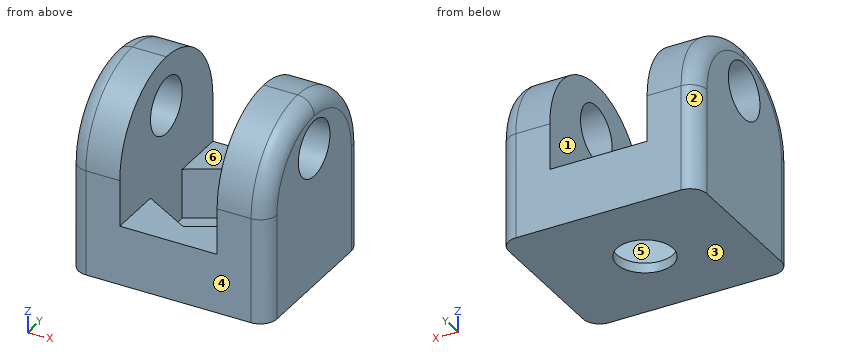
```python
from build123d import *

# Parameters (mm, degrees)
F0_R     = 1.7
F5_DEPTH = 0.6
F6_DEPTH = 3.6
F7_DEPTH = 11.4
F8_D     = 3.4
F8_DEPTH = 5
F8_START = 1
F8_TIP   = 1.0214630523
F9_D     = 3.4
F9_DEPTH = 5
F9_START = 1
F9_TIP   = 1.0214630523
F10_R    = 4.99999
F11_R    = 1


# Not quite as in the source:
# - a fillet or chamfer is up to 0.001 mm smaller than in the source, because OpenCascade refuses the exact size


with BuildPart() as f5:
    # F0 (on Top) → F5 (new body)
    with BuildSketch(Plane.XY):
        Polygon((0, 3.4), (-2.9444863729, 1.7), (-2.9444863729, -1.7), (0, -3.4), (2.9444863729, -1.7), (2.9444863729, 1.7), align=None)
        Circle(F0_R, mode=Mode.SUBTRACT)
    extrude(amount=F5_DEPTH)

    # F0 (on Top) → F6 (join)
    with BuildSketch(Plane.XY):
        Polygon((2.9444863729, 5), (-2.9444863729, 5), (-2.9444863729, 1.7), (0, 3.4), (2.9444863729, 1.7), align=None)
        Polygon((-2.9444863729, -1.7), (-2.9444863729, -5), (2.9444863729, -5), (2.9444863729, -1.7), (0, -3.4), align=None)
    extrude(amount=F6_DEPTH)

    # F0 (on Top) → F7 (join)
    with BuildSketch(Plane.XY):
        Polygon((-2.9444863729, 5), (-6, 5), (-6, -5), (-2.9444863729, -5), (-2.9444863729, -1.7), (-2.9444863729, 1.7), align=None)
        Polygon((6, 5), (2.9444863729, 5), (2.9444863729, 1.7), (2.9444863729, -1.7), (2.9444863729, -5), (6, -5), align=None)
    extrude(amount=F7_DEPTH)

    # F8
    # its depths count from where the whole tool has entered the part; down to there all is cleared
    with Locations(Plane(origin=(-7, 0, 0), x_dir=(0, 1, 0), z_dir=(-1, 0, 0)).offset(-F8_START)):
        with Locations((0, -8.4)):
            Hole(F8_D / 2, depth=F8_DEPTH)
            with Locations((0, 0, -(F8_DEPTH + F8_TIP / 2))):  # 118° drill point
                Cone(0, F8_D / 2, F8_TIP, mode=Mode.SUBTRACT)

    # F9
    # its depths count from where the whole tool has entered the part; down to there all is cleared
    with Locations(Plane.YZ.offset(7).offset(-F9_START)):
        with Locations((0, 8.4)):
            Hole(F9_D / 2, depth=F9_DEPTH)
            with Locations((0, 0, -(F9_DEPTH + F9_TIP / 2))):  # 118° drill point
                Cone(0, F9_D / 2, F9_TIP, mode=Mode.SUBTRACT)

    # F10 (radius 5 in the source; OpenCascade refuses exactly that, so slightly less here)
    f10_edges = [f5.edges().sort_by_distance(p)[0] for p in [
        (-4.472243, -5, 11.4),
        (-4.472243, 5, 11.4),
        (4.472243, 5, 11.4),
        (4.472243, -5, 11.4),
    ]]
    fillet(f10_edges, radius=F10_R)

    # F11
    f11_edges = [f5.edges().sort_by_distance(p)[0] for p in [
        (6, 3.535537, 9.935537),
        (-6, 3.535537, 9.935537),
    ]]
    fillet(f11_edges, radius=F11_R)


solid = f5.part
```
The listing builds one solid part. Answer for the finished solid, in the listing's coordinates (mm). Face numbers are marked on the shaded views. A direction names the side the tool comes from. Round coordinates to 2 decimals unless told otherwise and drop trailing zeros. Loops run counter-clockwise (first coordinate to the right, second up) from the corner with the lowest first, then second, coordinate; pieces in that order, holes last.
Q1. Section B-B, the plane z = 5.75 is taken. Determine the outline of the cut face in (x, y).
Q2. Section C-C, the plane x = -0.25 is taken. Determine the outline of the cut face in (y, z), then the cut area to 3 significant figures.
Q3. Find the intervals of material crossed by line 1 (X direction, y = 1.5, z = 1.5); line 2 (Y direction, x = 0, z = 0.35); line 3 (Z direction, x = 1.75, y = -1.75), in increasing order.
Q4. Section D-D, the plane z = 1 is taken. Determine the outline of the cut face in (x, y), then the cut area to 3 significant figures.
Q5. Given pin 1 Ø3.5 at (x, y) = (0.5, 3.5) entering from +Z, flat-ended and moving along its own axis, determine where the tip first touches the part or whether it passes through.
Q6. For a pull along X with two mould halves and no side action, classify the marked faces 1, 2 and 3 as released by +X, released by -X, zero draft, split by the parting line, or undercut.
Q7. Which of the six approach directions +Z, -Z, +X, -X, +Y, -Y give full straight-line access (tool end or side, diameter ignored) to the marked faces 4, 5 and 6?
Completed:
1. outline: (-6, -4) arc R1 ccw to (-5, -5) - (-2.94, -5) - (-2.94, 5) - (-5, 5) arc R1 ccw to (-6, 4) - close; (2.94, -5) - (5, -5) arc R1 ccw to (6, -4) - (6, 4) arc R1 ccw to (5, 5) - (2.94, 5) - close
2. outline: (-5, 0) - (-1.68, 0) - (-1.68, 0.6) - (-3.26, 0.6) - (-3.26, 3.6) - (-5, 3.6) - close; (1.68, 0) - (5, 0) - (5, 3.6) - (3.26, 3.6) - (3.26, 0.6) - (1.68, 0.6) - close
2. area: 14.4 mm2
3. line 1: x = -6 to -2.94, 2.94 to 6
3. line 2: y = -5 to -1.7, 1.7 to 5
3. line 3: z = 0 to 0.6
4. outline: (-6, -4) arc R1 ccw to (-5, -5) - (5, -5) arc R1 ccw to (6, -4) - (6, 4) arc R1 ccw to (5, 5) - (-5, 5) arc R1 ccw to (-6, 4) - close; hole (-2.94, -1.7) - (0, -3.4) - (2.94, -1.7) - (2.94, 1.7) - (0, 3.4) - (-2.94, 1.7) - close
4. area: 89.1 mm2
5. pin 1: stops at z = 3.6
6. face 1: undercut
6. face 2: released by -X
6. face 3: zero draft
7. face 4: +Z, -Z, +X, -X, -Y
7. face 5: +Z
7. face 6: +Z, +Y, -Y
